Geometry: see drawing. Coordinates: mm, zero at the bounding-box minimum. Give positions to 0.01 mm unless a question says otherwise; leave off trailing zeros. Order: outer loops, then holes, each group sorted by start corner. A loop starts at its lowest first (then second) coordinate and runs counter-clockwise, first axis right, second up. Notation, with made-up numbers: (49, -20.75) - (57, -20.75) arc R24 cw to (57, 1.25) - close; hole circle Ø8 at (11.25, -22). An arc over 180 degrees is marked (long way). One line per question, with ' | ' between items. Start each with the question number.
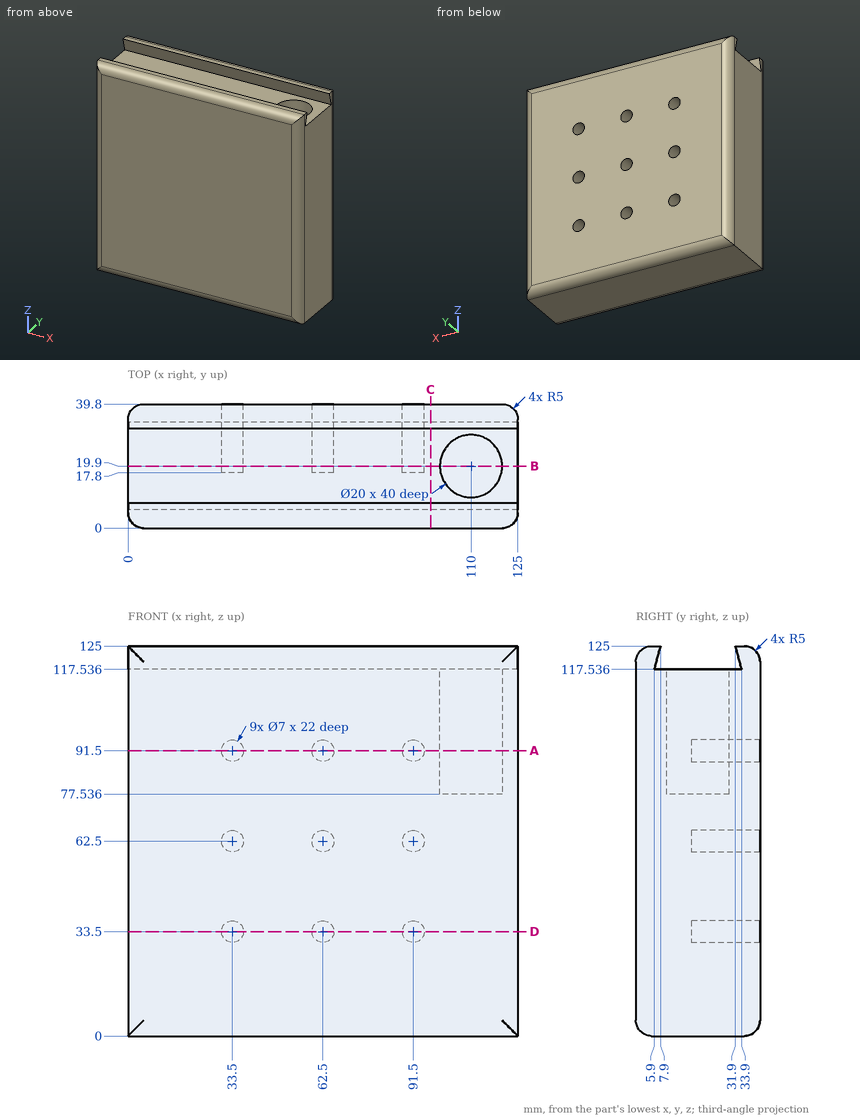
(1) Cut plane C-C, the plane x = 97. Return the cut outline in (y, z).
(2) Material intervals for line 1 along Z through (x, y) = (91, 24); line 2 along X through (y, z) = (31, 33); line 3 along X through (y, z) = (19, 94.5), sorted ascending. Write a range as from..to.
(3) Cut plane B-B, the plane y = 19.9. Give the number of separate pieces and of enclosed holes in the cut face, plus the area to 3 significant figures.
(4) Cut plane D-D, the plane z = 33.5. Return the cut outline in (x, y), plus the area to 3 significant figures.
(5) Contact query for flat-ended pins moving along their axis: P1, Ø6, axis at x = 18, y = 13.5, coming from the +Z side; P2, Ø3.5, axis at x = 33, z = 35, coming from the +Y side. Output: stop coordinate, or through.
(6) Cut plane A-A, the plane z = 91.5. Return the cut outline in (x, y), plus the area to 3 significant figures.
Results are:
1) outline: (0, 5) arc R5 ccw to (5, 0) - (34.8, 0) arc R5 ccw to (39.8, 5) - (39.8, 120) arc R5 ccw to (34.8, 125) - (31.9, 125) - (33.9, 117.54) - (5.9, 117.54) - (7.9, 125) - (5, 125) arc R5 ccw to (0, 120) - close
2) line 1: 0..30.04, 36.96..59.04, 65.96..88.04, 94.96..117.54 | line 2: 0..30.04, 36.96..59.04, 65.96..88.04, 94.96..125 | line 3: 0..31.7, 35.3..60.7, 64.3..89.7, 93.3..100.04, 119.96..125
3) separate pieces: 1 | enclosed holes: 9 | area: 13,500 mm2
4) outline: (0, 5) arc R5 ccw to (5, 0) - (120, 0) arc R5 ccw to (125, 5) - (125, 34.8) arc R5 ccw to (120, 39.8) - (95, 39.8) - (95, 17.8) - (88, 17.8) - (88, 39.8) - (66, 39.8) - (66, 17.8) - (59, 17.8) - (59, 39.8) - (37, 39.8) - (37, 17.8) - (30, 17.8) - (30, 39.8) - (5, 39.8) arc R5 ccw to (0, 34.8) - close | area: 4,490 mm2
5) P1: z = 117.54 | P2: y = 17.8
6) outline: (0, 5) arc R5 ccw to (5, 0) - (120, 0) arc R5 ccw to (125, 5) - (125, 34.8) arc R5 ccw to (120, 39.8) - (95, 39.8) - (95, 17.8) - (88, 17.8) - (88, 39.8) - (66, 39.8) - (66, 17.8) - (59, 17.8) - (59, 39.8) - (37, 39.8) - (37, 17.8) - (30, 17.8) - (30, 39.8) - (5, 39.8) arc R5 ccw to (0, 34.8) - close; hole circle Ø20 at (110, 19.9) | area: 4,180 mm2
